The listing builds one solid part. Answer for the finished solid, in the listing's coordinates (mm). Coordinates: 2 decimals unless noted, no trailing zeros. Order: outer loops, then holes, each group sorted by start corner. A loop starts at its lowest first (then second) coordinate and runs counter-clockwise, first axis right, second up. Notation, with made-up numbers: (-17.5, 52.25) -> (-11.5, 52.25) arc R10 ccw to (-11.5, 56.25) -> close; hole circle Ø1 at (81.5, 62.5). An arc over 180 degrees is marked (long way). Answer in a Markdown table with one row per item.
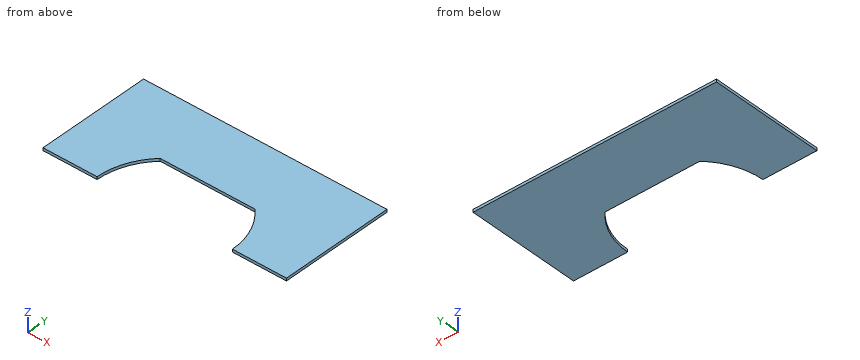
```python
from build123d import *

# Parameters (mm, degrees)
F1_DEPTH = 25.4
F2_DEPTH = 25.4


with BuildPart() as f1:
    # F0 (on Top) → F1 (new body)
    with BuildSketch(Plane.XY):
        with BuildLine():
            Line((0, 609.6), (-1143, 609.6))
            Line((-1143, 609.6), (-1143, 0))
            Line((-1143, 0), (-1143, -457.2))
            Line((-1143, -457.2), (-635, -457.2))
            ThreePointArc((-635, -457.2), (-585.441073, -211.265558), (-444.5, -3.719295))
            Line((-444.5, -3.719295), (444.5, -3.719295))
            ThreePointArc((444.5, -3.719295), (585.441073, -211.265558), (635, -457.2))
            Line((635, -457.2), (1143, -457.2))
            Line((1143, -457.2), (1143, 0))
            Line((1143, 0), (1143, 609.6))
            Line((1143, 609.6), (0, 609.6))
        make_face()
    extrude(amount=F1_DEPTH)

    # F0 (on Top) → F2 (join)
    with BuildSketch(Plane.XY):
        with BuildLine():
            Line((0, 609.6), (-1143, 609.6))
            Line((-1143, 609.6), (-1143, 0))
            Line((-1143, 0), (-1143, -457.2))
            Line((-1143, -457.2), (-635, -457.2))
            ThreePointArc((-635, -457.2), (-585.441073, -211.265558), (-444.5, -3.719295))
            Line((-444.5, -3.719295), (444.5, -3.719295))
            ThreePointArc((444.5, -3.719295), (585.441073, -211.265558), (635, -457.2))
            Line((635, -457.2), (1143, -457.2))
            Line((1143, -457.2), (1143, 0))
            Line((1143, 0), (1143, 609.6))
            Line((1143, 609.6), (0, 609.6))
        make_face()
    extrude(amount=F2_DEPTH)


solid = f1.part
```
(1) Find the intervals of material crossed by line 1 along Y through (x, z) = (-248, 4); line 2 along X through (y, z) = (-318, 22.5); line 3 along X through (y, z) = (-29.5, 10.5), in increasing order. Write a range as from..to.
Check values:
| item | result |
|---|---|
| line 1 | -3.72..609.6 |
| line 2 | -1143..-619.55, 619.55..1143 |
| line 3 | -1143..-469.36, 469.36..1143 |
(2) A cutting plane is placed at C-C, the plane x = 38.5. Determine the outline of the cut face in (y, z), then the cut area to 3 significant figures.
Check values:
| item | result |
|---|---|
| outline | (-3.72, 0) -> (609.6, 0) -> (609.6, 25.4) -> (-3.72, 25.4) -> close |
| area | 15,600 mm² |
(3) A cutting plane is placed at A-A, the plane y = -187. Determine the outline of the cut face in (x, z).
Check values:
| item | result |
|---|---|
| outline | (-1143, 0) -> (-574.65, 0) -> (-574.65, 25.4) -> (-1143, 25.4) -> close; (574.65, 0) -> (1143, 0) -> (1143, 25.4) -> (574.65, 25.4) -> close |
(4) A cutting plane is placed at B-B, the plane z = 6.25. Determine the outline of the cut face in (x, y), then the cut area to 3 significant figures.
Check values:
| item | result |
|---|---|
| outline | (-1143, -457.2) -> (-635, -457.2) arc R635 cw to (-444.5, -3.72) -> (444.5, -3.72) arc R635 cw to (635, -457.2) -> (1143, -457.2) -> (1143, 609.6) -> (-1143, 609.6) -> close |
| area | 1,920,000 mm² |
(5) A cutting plane is placed at D-D, the plane y = -319. Determine the outline of the cut face in (x, z).
Check values:
| item | result |
|---|---|
| outline | (-1143, 0) -> (-619.78, 0) -> (-619.78, 25.4) -> (-1143, 25.4) -> close; (619.78, 0) -> (1143, 0) -> (1143, 25.4) -> (619.78, 25.4) -> close |
